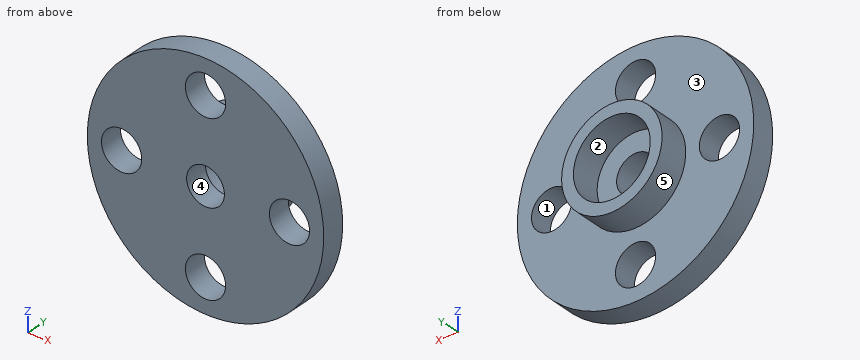
Autodesk Inventor part; units mm, degrees
ref_plane "YZ Plane" through (0, 0, 0) normal (1, 0, 0) x (0, 1, 0)
ref_plane "XZ Plane" through (0, 0, 0) normal (0, 1, 0) x (-1, 0, 0)
ref_plane "XY Plane" through (0, 0, 0) normal (0, 0, 1) x (1, 0, 0)
sketch "Эскиз1" plane through (0, 0, 0) normal (0, 1, 0) x (-1, 0, 0)
  circle A0 centre (0, 0) radius 10
  circle A1 centre (0, 0) radius 1.6
  circle A2 centre (0, 7.1) radius 1.7
  circle A3 centre (-7.1, 0) radius 1.7
  circle A4 centre (0, -7.1) radius 1.7
  circle A5 centre (7.1, 0) radius 1.7
  dimension "d0" = 20
  dimension "d1" = 3.2
  dimension "d2" = 3.4
  dimension "d3" = 1.2
  dimension "d6" = 360
extrude "Выдавливание1" add sketch "Эскиз1" along normal blind 2
sketch "Эскиз2" plane through (0, 2, 0) normal (0, 1, 0) x (1, 0, 0)
  circle A0 centre (0, 0) radius 1.6
  circle A1 centre (0, 0) radius 4.25
  circle A2 centre (0, 0) radius 3.25
  dimension "d10" = 8.5
  dimension "d11" = 6.5
extrude "Выдавливание2" add sketch "Эскиз2" along normal blind 2.5 contours A1
properties part number "Servo krepej"
Input: part model. Units: mm. Frame: model coordinates. Face numbers are marked on the shaded views. A direction names the side the tool comes from. Give positions to 0.01 mm unless a question says otherwise; leave off trailing zeros. Write each loop counter-clockwise with the first axis right and the second up, starting at its lowest first coordinate (ties: lowest second). Pieces come first, ordered by that corner, then holes.
Q1. Section C-C, the plane y = 1.4. Output: boundary loops of the cut face in (x, z).
Q2. Pull-direction query (X, two-part tool) for the marked faces 3, 4 and 5; classes: pulls with the +X half, pulls with the -X half, needs draft (parallel to the pull), parting line crosses it, or undercut.
Q3. Section B-B, the plane x = 0. Output: boundary loops of the cut face in (y, z).
Q4. First-contact query: P1, Ø3, axis at x = 0, z = -7.1, coming from the -Y side; P2, Ø2, axis at x = 7.5, y = 2.5, coming from the -Z side; P3, Ø6, axis at x = 0, z = 0, coming from the +Y side; P4, Ø2, axis at x = -2, y = 2.5, coming from the -Z side. Flat tips, straight axial feed; report the tip coordinate or a pass-through.
Q5. Set-up query: the marked faces 1 and 2. Return all of +Z, -Z, +X, -X, +Y, -Y with unobstructed straight access to the full face (end or side cutting, diameter ignored); none if empty.
Q6. Material intervals for probe 1 along Z at (x, y) = (0, 1); probe 2 along X at (y, z) = (3.25, 0); probe 3 along Z at (x, y) = (-1.25, 1), sorted ascending.
Q7. Section D-D, the plane x = 7. Output: boundary loops of the cut face in (y, z), plus the area to 3 significant figures.
Q8. Section A-A, the plane z = 0. Output: boundary loops of the cut face in (x, y).
Filled in:
1. outline: circle Ø20 at (0, 0); hole circle Ø3.4 at (-7.1, 0); hole circle Ø3.4 at (0, -7.1); hole circle Ø3.4 at (0, 7.1); hole circle Ø3.2 at (0, 0); hole circle Ø3.4 at (7.1, 0)
2. face 3: needs draft
2. face 4: undercut
2. face 5: parting line crosses it
3. outline: (0, -10) - (2, -10) - (2, -8.8) - (0, -8.8) - close; (0, -5.4) - (2, -5.4) - (2, -4.25) - (4.5, -4.25) - (4.5, -3.25) - (2, -3.25) - (2, -1.6) - (0, -1.6) - close; (0, 1.6) - (2, 1.6) - (2, 3.25) - (4.5, 3.25) - (4.5, 4.25) - (2, 4.25) - (2, 5.4) - (0, 5.4) - close; (0, 8.8) - (2, 8.8) - (2, 10) - (0, 10) - close
4. P1: passes through
4. P2: stops at z = -7.48
4. P3: stops at y = 2
4. P4: stops at z = -9.94
5. face 1: +Y, -Y
5. face 2: +Y
6. probe 1: z = -10 to -8.8, -5.4 to -1.6, 1.6 to 5.4, 8.8 to 10
6. probe 2: x = -4.25 to -3.25, 3.25 to 4.25
6. probe 3: z = -9.92 to -8.25, -5.95 to -1, 1 to 5.95, 8.25 to 9.92
7. outline: (0, -7.14) - (2, -7.14) - (2, -1.7) - (0, -1.7) - close; (0, 1.7) - (2, 1.7) - (2, 7.14) - (0, 7.14) - close
7. area: 21.8 mm2
8. outline: (-10, 0) - (-8.8, 0) - (-8.8, 2) - (-10, 2) - close; (-5.4, 0) - (-1.6, 0) - (-1.6, 2) - (-3.25, 2) - (-3.25, 4.5) - (-4.25, 4.5) - (-4.25, 2) - (-5.4, 2) - close; (1.6, 0) - (5.4, 0) - (5.4, 2) - (4.25, 2) - (4.25, 4.5) - (3.25, 4.5) - (3.25, 2) - (1.6, 2) - close; (8.8, 0) - (10, 0) - (10, 2) - (8.8, 2) - close
